Here's how the part is built. I have some questions about the finished solid (model axes, mm). A direction names the side the tool comes from. Coordinates: 2 decimals unless noted, no trailing zeros. Write each loop counter-clockwise with the first axis right and the second up, starting at its lowest first coordinate (ties: lowest second). Pieces come first, ordered by that corner, then holes. Notation, with made-up numbers: (64, -18.75) -> (73, -18.75) arc R19 cw to (73, -10.75) -> close; hole circle Ø9 at (-4.5, 68). An arc over 180 degrees is marked (long way). Put each result on its own line as item: value.
Autodesk Inventor part; units mm, degrees
ref_plane "YZ Plane" through (0, 0, 0) normal (1, 0, 0) x (0, 1, 0)
ref_plane "XZ Plane" through (0, 0, 0) normal (0, 1, 0) x (-1, 0, 0)
ref_plane "XY Plane" through (0, 0, 0) normal (0, 0, 1) x (1, 0, 0)
sketch "Sketch1" plane through (0, 0, 0) normal (0, 1, 0) x (-1, 0, 0)
  line L0 (-9, 0) -> (9, 0)
  arc A0 (-9, 0) -> (-10, -1) centre (-9, -1) ccw
  line L1 (-10, -1) -> (-10, -6.1474)
  arc A1 (-10, -6.1474) -> (-9.9358, -6.5) centre (-9, -6.1474) ccw
  line L2 (-9.9358, -6.5) -> (-7.0184, -14.2433)
  arc A2 (-7.0184, -14.2433) -> (7.0184, -14.2433) centre (0, -11.599) ccw
  line L3 (7.0184, -14.2433) -> (9.9358, -6.5)
  arc A3 (9.9358, -6.5) -> (10, -6.1474) centre (9, -6.1474) ccw
  line L4 (10, -6.1474) -> (10, -1)
  arc A4 (10, -1) -> (9, 0) centre (9, -1) ccw
  line L5 (9, 1.5) -> (-9, 1.5)
  arc A5 (-9, 1.5) -> (-11.5, -1) centre (-9, -1) ccw
  line L6 (-11.5, -1) -> (-11.5, -6.1474)
  arc A6 (-11.5, -6.1474) -> (-11.3395, -7.0289) centre (-9, -6.1474) ccw
  line L7 (-11.3395, -7.0289) -> (-8.4221, -14.7721)
  arc A7 (-8.4221, -14.7721) -> (8.4221, -14.7721) centre (0, -11.599) ccw
  line L8 (8.4221, -14.7721) -> (11.3395, -7.0289)
  arc A8 (11.3395, -7.0289) -> (11.5, -6.1474) centre (9, -6.1474) ccw
  line L9 (11.5, -6.1474) -> (11.5, -1)
  arc A9 (11.5, -1) -> (9, 1.5) centre (9, -1) ccw
  point P0 (0, 0)
  point P1 (0, 0)
  dimension "d0" = 18
  dimension "d1" = 6.5
  dimension "d2" = 1
  dimension "d3" = 1
  dimension "d4" = 9
  dimension "d5" = 7.5
  dimension "d6" = 1
  dimension "d7" = 1
  dimension "d8" = 11.599
  dimension "d9" = 1.5
extrude "Extrusion1" add sketch "Sketch1" along normal blind 2
fillet "Fillet1" radius 0.3 40 edges at (10.7678, 2, 0.7678) (11.5, 2, -3.5737) (11.4595, 2, -6.5954) (9.8808, 2, -10.9005) (0, 2, -20.599) (-9.8808, 2, -10.9005) (-11.4595, 2, -6.5954) (-11.5, 2, -3.5737) (-10.7678, 2, 0.7678) (0, 2, 1.5) (10.7678, 0, 0.7678) (11.5, 0, -3.5737) (11.4595, 0, -6.5954) (9.8808, 0, -10.9005) (0, 0, -20.599) (-9.8808, 0, -10.9005) (-11.4595, 0, -6.5954) (-11.5, 0, -3.5737) (-10.7678, 0, 0.7678) (0, 0, 1.5) (-9.7071, 2, -0.2929) (-10, 2, -3.5737) (-9.9838, 2, -6.3266) (-8.4771, 2, -10.3716) (0, 2, -19.099) (8.4771, 2, -10.3716) (9.9838, 2, -6.3266) (10, 2, -3.5737) (9.7071, 2, -0.2929) (0, 2, 0) (9.7071, 0, -0.2929) (10, 0, -3.5737) (9.9838, 0, -6.3266) (8.4771, 0, -10.3716) (0, 0, -19.099) (-8.4771, 0, -10.3716) (-9.9838, 0, -6.3266) (-10, 0, -3.5737) (-9.7071, 0, -0.2929) (0, 0, 0)
equation "\"d3\" = d2"
equation "\"d6\" = d3"
equation "\"d7\" = d6"
properties part number "y_carryage_bearing_zip_tie" material "ABS Plastic"
Item 1: Imagine slicing it at B-B on y = 1. Write out the boundary of the cut face in (x, z), then the cut area to 3 significant figures.
Output:
outline: (-11.5, -6.15) arc R2.5 ccw to (-11.34, -7.03) -> (-8.42, -14.77) arc R9 ccw to (8.42, -14.77) -> (11.34, -7.03) arc R2.5 ccw to (11.5, -6.15) -> (11.5, -1) arc R2.5 ccw to (9, 1.5) -> (-9, 1.5) arc R2.5 ccw to (-11.5, -1) -> close; hole (-10, -6.15) arc R1 ccw to (-9.94, -6.5) -> (-7.02, -14.24) arc R7.5 ccw to (7.02, -14.24) -> (9.94, -6.5) arc R1 ccw to (10, -6.15) -> (10, -1) arc R1 ccw to (9, 0) -> (-9, 0) arc R1 ccw to (-10, -1) -> close
area: 107 mm²
Item 2: Which directions (+Z, -Z, +X, -X, +Y, -Y) give clear straight access to the entire face, cutting with the end or side of a thin tool? Please do faces 4 (the cylindrical face through (-9.82, 0.09, -10.82)), 5 (the cylindrical face through (-8.582, 0.086, -10.349)), 6 (the cylindrical face through (8.537, 1.91, -10.456)), 7 (the flat face through (0, 1, 0)).
Output:
face 4: -Z, -X, -Y
face 5: -Y
face 6: +Y
face 7: +Y, -Y
Item 3: If we mould it in two halves opening along X, with no side actions, what happens to faces 1 (the flat face through (11.5, 1, -4)), 2 (the flat face through (-11.5, 1, -4)), 3 (the cylindrical face through (9.715, 0.99, -0.301))? For each: released by +X, released by -X, zero draft, split by the parting line, or undercut.
Output:
face 1: released by +X
face 2: released by -X
face 3: undercut
Item 4: Please list where these lines run through material, in increasing order: line 1 along X through (y, z) = (0.35, -1.25); line 2 along X through (y, z) = (1.05, -16.25); line 3 along Z through (x, y) = (-4.5, 1.3). Write a range as from..to.
Output:
line 1: x = -11.5..-10, 10..11.5
line 2: x = -7.71..-5.88, 5.88..7.71
line 3: z = -19.39..-17.6, 0..1.5
Item 5: Imagine slicing it at A-A on z = -2.5. Write out the boundary of the cut face in (x, y).
Output:
outline: (-11.5, 0.3) arc R0.3 ccw to (-11.2, 0) -> (-10.3, 0) arc R0.3 ccw to (-10, 0.3) -> (-10, 1.7) arc R0.3 ccw to (-10.3, 2) -> (-11.2, 2) arc R0.3 ccw to (-11.5, 1.7) -> close; (10, 0.3) arc R0.3 ccw to (10.3, 0) -> (11.2, 0) arc R0.3 ccw to (11.5, 0.3) -> (11.5, 1.7) arc R0.3 ccw to (11.2, 2) -> (10.3, 2) arc R0.3 ccw to (10, 1.7) -> close
Item 6: For P1, Ø1.1, axis at x = -4.5, y = 1, coming from the -Z side, with a flat end and sliding along its axis, tell me the tip position at first contact or that it passes through.
Output:
P1: stops at z = -19.69
